```python
from build123d import *

# Parameters (mm, degrees)
IZIM1_W                     = 20
IZIM1_H                     = 20
Y_KSEKLIK_EKSTR_ZYON1_DEPTH = 160
IZIM13_R                    = 1.5
KES_EKSTR_ZYON1_DEPTH       = 10
KES_EKSTR_ZYON2_START       = -10
IZIM15_R                    = 1.5
KES_EKSTR_ZYON2_DEPTH       = 10
IZIM18_R                    = 1.5
KES_EKSTR_ZYON3_DEPTH       = 10
IZIM20_R                    = 1.5
KES_EKSTR_ZYON4_DEPTH       = 10
SKETCH1_R                   = 1.5
CUT_EXTRUDE1_DEPTH          = 10
SKETCH2_R                   = 1.5
CUT_EXTRUDE2_DEPTH          = 10


with BuildPart() as part:
    # Çizim1 → Yükseklik-Ekstrüzyon1 (new body)
    with BuildSketch(Plane.XY):
        with Locations((10, 10)):
            Rectangle(IZIM1_W, IZIM1_H)
    extrude(amount=Y_KSEKLIK_EKSTR_ZYON1_DEPTH)

    # Çizim13 → Kes-Ekstrüzyon1 (cut)
    with BuildSketch(Plane.XY.offset(160)):
        with Locations((14, 6)):
            Circle(IZIM13_R)
        with Locations((6, 14)):
            Circle(IZIM13_R)
    extrude(amount=-KES_EKSTR_ZYON1_DEPTH, mode=Mode.SUBTRACT)

    # Çizim15 → Kes-Ekstrüzyon2 (cut)
    with BuildSketch(Plane(origin=(0, 0, 0), x_dir=(-1, 0, 0), z_dir=(0, 0, -1)).offset(KES_EKSTR_ZYON2_START)):
        with Locations(Location((-14, 6, 0), (0, 0, 180))):
            Circle(IZIM15_R)
        with Locations(Location((-6, 14, 0), (0, 0, 180))):
            Circle(IZIM15_R)
    extrude(amount=KES_EKSTR_ZYON2_DEPTH, mode=Mode.SUBTRACT)

    # Çizim18 → Kes-Ekstrüzyon3 (cut)
    with BuildSketch(Plane(origin=(20, 0, 0), x_dir=(0, 0, -1), z_dir=(1, 0, 0))):
        with Locations((-10, 13)):
            Circle(IZIM18_R)
        with Locations((-150, 13)):
            Circle(IZIM18_R)
    extrude(amount=-KES_EKSTR_ZYON3_DEPTH, mode=Mode.SUBTRACT)

    # Çizim20 → Kes-Ekstrüzyon4 (cut)
    with BuildSketch(Plane.XZ):
        with Locations(Location((7, 10, 0), (0, 0, 270))):
            Circle(IZIM20_R)
        with Locations(Location((7, 150, 0), (0, 0, 270))):
            Circle(IZIM20_R)
    extrude(amount=-KES_EKSTR_ZYON4_DEPTH, mode=Mode.SUBTRACT)

    # Sketch1 → Cut-Extrude1 (cut)
    with BuildSketch(Plane(origin=(0, 20, 0), x_dir=(1, 0, 0), z_dir=(0, 1, 0))):
        with Locations(Location((13, -20, 0), (0, 0, 270))):
            Circle(SKETCH1_R)
        with Locations(Location((13, -80, 0), (0, 0, 270))):
            Circle(SKETCH1_R)
        with Locations(Location((13, -140, 0), (0, 0, 270))):
            Circle(SKETCH1_R)
    extrude(amount=-CUT_EXTRUDE1_DEPTH, mode=Mode.SUBTRACT)

    # Sketch2 → Cut-Extrude2 (cut)
    with BuildSketch(Plane.ZY):
        with Locations((20, 7)):
            Circle(SKETCH2_R)
        with Locations((80, 7)):
            Circle(SKETCH2_R)
        with Locations((140, 7)):
            Circle(SKETCH2_R)
    extrude(amount=-CUT_EXTRUDE2_DEPTH, mode=Mode.SUBTRACT)


solid = part.part
```
The listing builds one solid part. Answer for the finished solid, in the listing's coordinates (mm). A direction names the side the tool comes from. Coordinates: 2 decimals unless noted, no trailing zeros. Loops run counter-clockwise (first coordinate to the right, second up) from the corner with the lowest first, then second, coordinate; pieces in that order, holes last. Notation, with made-up numbers: M -6,89.25 L -1,89.25 A31 cw -1,121.25 Z; hole C 58.5,-8 d4. An arc over 180 degrees is marked long. Answer as a JSON object with one key per item and string values. Group by question number.
Item 1: Determine the mould class of faces 1 (the face through (10, 13, 150)), 2 (the face through (15.07, 13.07, 151.5)), 3 (the face through (13.07, 15.07, 138.5)) for opening direction X: +X half, -X half, draft (parallel to the pull), parting line (faces both ways), or undercut.
Item 2: Section A-A (z = 20) is taken. Write down the section's boundary in (x, y), and give its area (3 significant figures).
Item 3: Which of the six approach directions +Z, -Z, +X, -X, +Y, -Y give full straight-line access (tool end or side, diameter ignored) to faces 4 (the face through (12.5, 5.93, 5.07)), 5 (the face through (6, 14, 150)), 6 (the face through (13.07, 15.07, 18.5))?
Item 4: Consider L1, parallel to Y at x = 7.5, z = 20; L2, parallel to Y at x = 6, z = 7.75; L3, parallel to X at y = 16.5, z = 20. Determine where each line is inside the solid, lowest interval first.
Item 5: Each of these flat-tipped pins is pushed along its axis until it touches: P1, Ø1.5, axis at y = 7, z = 80.5, coming from the -X side; P2, Ø2.5, axis at x = 7, z = 10, coming from the -Y side; P3, Ø0.9, axis at x = 13, z = 140, coming from the +Y side; P4, Ø4, axis at y = 18, z = 67.5, coming from the -X side. Where does it stop, or does it pass through?
Solved:
{
 "1": {"face 1": "+X half", "face 2": "draft", "face 3": "undercut"},
 "2": {"outline": "M 0,0 L 20,0 L 20,20 L 14.5,20 L 14.5,10 L 11.5,10 L 11.5,20 L 0,20 L 0,8.5 L 10,8.5 L 10,5.5 L 0,5.5 Z", "area": "340 mm2"},
 "3": {"face 4": "-Z", "face 5": "+Z", "face 6": "+Y"},
 "4": {"L1": "y = 0 to 5.5, 8.5 to 20", "L2": "y = 0 to 12.5, 15.5 to 20", "L3": "x = 0 to 11.5, 14.5 to 20"},
 "5": {"P1": "stops at x = 10", "P2": "stops at y = 10", "P3": "stops at y = 10", "P4": "stops at x = 0"}
}
